```python
from build123d import *

# Parameters (mm, degrees)
F0_R          = 6.35
F1_DEPTH      = 50.8
F2_R          = 6.35
F3_DEPTH      = 17.78
F4_R          = 8.89
F4_R_2        = 6.35
F5_DEPTH      = 5.08
F6_W          = 12.7
F6_H          = 6.35
F7_DEPTH      = 12.7
F7_DEPTH_BACK = 25.4
F8_R          = 1.905
F9_DEPTH      = 12.7


with BuildPart() as f1:
    # F0 (on Right) → F1 (new body)
    with BuildSketch(Plane.YZ):
        with BuildLine():
            Line((-7.428396, 34.981928), (-20.128396, 34.981928))
            ThreePointArc((-20.128396, 34.981928), (-29.108653, 31.262184), (-32.828396, 22.281928))
            Line((-32.828396, 22.281928), (-32.828396, 3.089348))
            ThreePointArc((-32.828396, 3.089348), (-33.572345, 1.293297), (-35.368396, 0.549348))
            Line((-35.368396, 0.549348), (-48.068396, 0.549348))
            ThreePointArc((-48.068396, 0.549348), (-49.864448, -0.194601), (-50.608396, -1.990652))
            Line((-50.608396, -1.990652), (-50.608396, -11.728213))
            ThreePointArc((-50.608396, -11.728213), (-51.352345, -13.524265), (-53.148396, -14.268213))
            Line((-53.148396, -14.268213), (-68.388396, -14.268213))
            ThreePointArc((-68.388396, -14.268213), (-70.184448, -13.524265), (-70.928396, -11.728213))
            Line((-70.928396, -11.728213), (-70.928396, 10.851928))
            ThreePointArc((-70.928396, 10.851928), (-72.788268, 15.342056), (-77.278396, 17.201928))
            Line((-77.278396, 17.201928), (-139.508396, 17.201928))
            Line((-139.508396, 17.201928), (-140.272923, 17.201928))
            ThreePointArc((-140.272923, 17.201928), (-144.931511, 15.167024), (-146.604342, 10.366514))
            Line((-146.604342, 10.366514), (-142.028059, -49.323486))
            ThreePointArc((-142.028059, -49.323486), (-140.011736, -53.49666), (-135.69664, -55.188072))
            Line((-135.69664, -55.188072), (-134.428396, -55.188072))
            Line((-134.428396, -55.188072), (-101.488806, -50.828371))
            Line((-101.488806, -50.828371), (-66.222131, -48.624206))
            Line((-66.222131, -48.624206), (-30.514626, -50.828371))
            Line((-30.514626, -50.828371), (-7.428396, -55.188072))
            ThreePointArc((-7.428396, -55.188072), (1.55186, -51.468328), (5.271604, -42.488072))
            Line((5.271604, -42.488072), (5.271604, 22.281928))
            ThreePointArc((5.271604, 22.281928), (1.55186, 31.262184), (-7.428396, 34.981928))
        make_face()
        with Locations((-123.933047, -36.138072)):
            Circle(F0_R, mode=Mode.SUBTRACT)
        with Locations((-13.778396, -29.788072)):
            Circle(F0_R, mode=Mode.SUBTRACT)
    extrude(amount=F1_DEPTH)

    # F2 (on face) → F3 (join)
    with BuildSketch(Plane.XY.offset(17.201928)):
        with Locations((38.1, -108.77391)):
            Circle(F2_R)
    extrude(amount=F3_DEPTH)

    # F4 (on face) → F5 (join)
    with BuildSketch(Plane.XY.offset(34.981928)):
        with Locations((38.1, -108.77391)):
            Circle(F4_R)
        with Locations((38.1, -108.77391)):
            Circle(F4_R_2, mode=Mode.SUBTRACT)
        with Locations((38.1, -108.77391)):
            Circle(F4_R_2)
    extrude(amount=F5_DEPTH)

    # F6 (on face) → F7 (join, two sides)
    with BuildSketch(Plane(origin=(0, 5.271604, 0), x_dir=(-1, 0, 0), z_dir=(0, 1, 0))) as f7_sk:
        with Locations((-25.4, -45.663072)):
            Rectangle(F6_W, F6_H)
    extrude(amount=F7_DEPTH)
    extrude(f7_sk.sketch, amount=-F7_DEPTH_BACK)

    # F8 (on face) → F9 (cut)
    with BuildSketch(Plane.XY.offset(-42.488072)):
        with Locations((25.4, 11.621604)):
            Circle(F8_R)
    extrude(amount=-F9_DEPTH, mode=Mode.SUBTRACT)


solid = f1.part
```
CAD build for the part. Positions are in the model's coordinates, mm. A direction names the side the tool comes from. Round coordinates to 2 decimals unless told otherwise and drop trailing zeros. Order: outer loops, then holes, each group sorted by start corner. A loop starts at its lowest first (then second) coordinate and runs counter-clockwise, first axis right, second up. Notation, with made-up numbers: (-11, 26) - (6, 26) arc R29 ccw to (6, 50) - close; hole circle Ø5 at (65.5, 19.25). An arc over 180 degrees is marked (long way). Answer in a Markdown table with one row per item. Add a question column.
(1) Mould opens along Y. For faces 4 (the face through (50.8, -72, -19)), 5 (the face through (25.044, 1.65, 31.163)), 6 (the face through (25.044, -72.739, 15.292)) say: +Y half, -Y half, draft (parallel to the pull), parting line (faces both ways), or undercut.
(2) Band-saw the part on D-D on y = -125. List the corners of the cut face in (x, z).
(3) Drop flat-ended pins along their axis: pin 1 Ø8 at (x, z) = (28, 22) entering from +Y; pin 2 Ø6 at (x, y) = (36, -83) entering from +Z; pin 3 Ø10 at (x, y) = (11.5, -110) entering from -Z. Give the stop position or say it passes through.
(4) Band-saw the part on A-A on x = 25.4. Count the separate pieces of the cut face and the enclosed holes in it, and give its area (3 significant figures).
(5) Probe L1, parallel to Y at x = 5, z = -5.5; L2, parallel to Y at x = 16, z = -39; L3, parallel to X at y = -109, z = 21. List the from-to ranges inside material, lowest first. Write a range as [from, to].
(6) 3-axis set-ups, long thin cutter, end or side, ignore diameter. For faces 1 (the face through (25, -42, 0.549)), 2 (the face through (27, 10, -42.488)), 3 (the face through (25.04, -48.62, -49.71)): which of +Z, -Z, +X, -X, +Y, -Y reach the whole face in a straight line?
(7) Band-saw the part on C-C on z = 7. List the corners of the cut face in (x, y).
Data:
| question | item | result |
|---|---|---|
| 1 | face 4 | draft |
| 1 | face 5 | +Y half |
| 1 | face 6 | undercut |
| 2 | outline | (0, -53.94) - (50.8, -53.94) - (50.8, -42.4) - (0, -42.4) - close; (0, -29.88) - (50.8, -29.88) - (50.8, 17.2) - (0, 17.2) - close |
| 3 | pin 1 | stops at y = 5.27 |
| 3 | pin 2 | stops at z = 17.2 |
| 3 | pin 3 | stops at z = -52.62 |
| 4 | separate pieces | 2 |
| 4 | enclosed holes | 2 |
| 4 | area | 9,740 mm^2 |
| 5 | L1 | y = [-145.39, -70.93], [-50.61, 5.27] |
| 5 | L2 | y = [-142.82, -129.6], [-118.26, 5.27] |
| 5 | L3 | x = [31.75, 44.45] |
| 6 | face 1 | +Z, +X, -X |
| 6 | face 2 | +Z, +X, -X, +Y |
| 6 | face 3 | -Z, +X, -X |
| 7 | outline | (0, -146.35) - (50.8, -146.35) - (50.8, -70.93) - (0, -70.93) - close; (0, -32.83) - (50.8, -32.83) - (50.8, 5.27) - (0, 5.27) - close |
